Geometry: see drawing. Coordinates: mm, zero at the bounding-box minimum. Coordinates: 2 decimals unless noted, no trailing zeros. Order: outer loops, then holes, each group sorted by start corner. A loop starts at its lowest first (then second) coordinate and runs counter-clockwise, first axis right, second up.
Item 1: Section C-C on z = 3.25. Return the cut outline in (x, y).
Item 2: Mould query, pull axis Y, two halves, no side actions, for the marked faces 1, 2 and 3. Classes: released by +Y, released by -Y, zero draft, split by the parting line, or undercut.
Item 3: Section D-D on y = 1.5. Return the cut outline in (x, z).
Item 4: Ray query, line 1 (Y direction, x = 5.5, z = 7.8); line 2 (Y direction, x = 5.5, z = 3.5); line 3 (Z direction, x = 4.5, y = 5). Return the intervals inside material, ascending.
Item 5: Contact query for flat-ended pins moving along their axis: P1, Ø1, axis at x = 2, z = 7.5, coming from the -Y side; P2, Ø2, axis at y = 8, z = 1.5, coming from the +X side; P3, Ø2, axis at x = 7, z = 6, coming from the +Y side. Output: stop coordinate, or through.
Item 6: Section A-A on y = 5.5. Return the cut outline in (x, z).
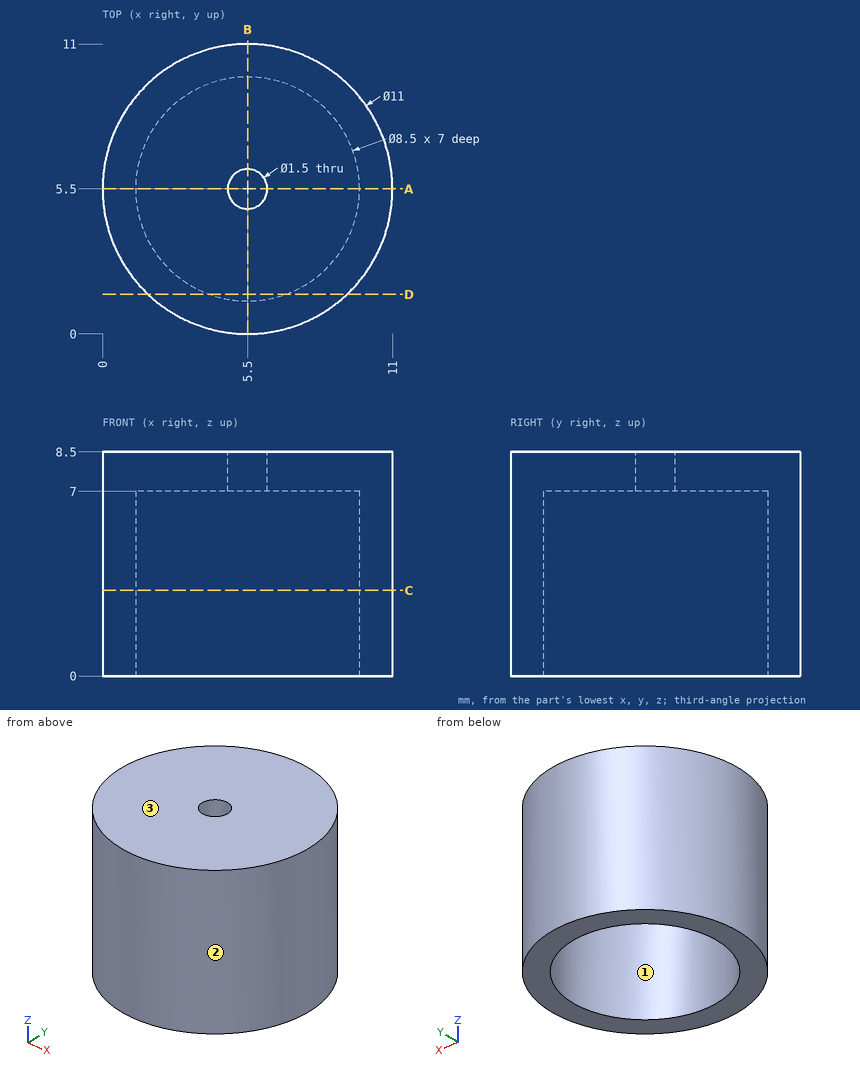
Answer list:
1. outline: circle Ø11 at (5.5, 5.5); hole circle Ø8.5 at (5.5, 5.5)
2. face 1: undercut
2. face 2: split by the parting line
2. face 3: zero draft
3. outline: (1.73, 0) - (4.06, 0) - (4.06, 7) - (6.94, 7) - (6.94, 0) - (9.27, 0) - (9.27, 8.5) - (1.73, 8.5) - close
4. line 1: y = 0 to 4.75, 6.25 to 11
4. line 2: y = 0 to 1.25, 9.75 to 11
4. line 3: z = 7 to 8.5
5. P1: stops at y = 0.89
5. P2: stops at x = 10.79
5. P3: stops at y = 10.98
6. outline: (0, 0) - (1.25, 0) - (1.25, 7) - (4.75, 7) - (4.75, 8.5) - (0, 8.5) - close; (6.25, 7) - (9.75, 7) - (9.75, 0) - (11, 0) - (11, 8.5) - (6.25, 8.5) - close
